The model under review builds one solid part; all positions refer to its coordinate system, in mm. A direction names the side the tool comes from. Round coordinates to 2 decimals unless told otherwise and drop trailing zeros. Loops run counter-clockwise (first coordinate to the right, second up) from the corner with the lowest first, then second, coordinate; pieces in that order, holes last. Notation, with made-up numbers: (74.5, -30.75) -> (110.5, -30.75) arc R14 ccw to (110.5, -11.75) -> close; hole circle Ø3 at (-32.75, 54.5). An arc over 180 degrees is marked (long way). Write each question's results on one line, items separated by ' | '. Start each with the question number.
Item 1: We need section B-B (z = -2). Give the boundary of the cut face in (x, y), and give its area (3 significant figures).
Item 2: Tool access review of faces 1 (the flat face through (84, 6, 0)), 2 (the flat face through (-36, 6, 0)): name each direction out of +Z, -Z, +X, -X, +Y, -Y from which nothing blocks a thin tool from reaching the whole face with its end or side.
Item 3: We need section C-C (x = 15). Give the boundary of the cut face in (y, z), and give its area (3 significant figures).
Item 4: For L1, parallel to X at y = 6.5, z = 18; L2, parallel to X at y = 2.25, z = -20.5; L3, parallel to Z at x = 13, y = 4.5, list the stretches that pass through material, from the lowest coordinate up. Write a range as from..to.
Item 5: Mouldability with a two-part tool opening along X and no side actions: class faces 3 (the flat face through (-1, 6, -23)), 4 (the flat face through (-1, 12, -24)), 5 (the flat face through (-84, 6, 0)), 6 (the cylindrical face through (-73.77, 5.92, 24.96)) as pulls with the +X half, pulls with the -X half, needs draft (parallel to the pull), parting line crosses it, or undercut.
Item 6: We need section A-A (x = -72). Give the boundary of the cut face in (y, z), and give its area (3 significant figures).
Item 7: We need section D-D (y = 4). Give the boundary of the cut face in (x, z).
from build123d import *

# Parameters (mm, degrees)
SKETCH1_W                  = 168
SKETCH1_H                  = 70
SKETCH1_R                  = 4.25
SKETCH1_W_2                = 72
SKETCH1_H_2                = 46
BRIDGE_CLAMP_EXTRUDE_DEPTH = 12


with BuildPart() as part:
    # Sketch1 → Bridge_Clamp_Extrude (new body)
    with BuildSketch(Plane(origin=(0, 0, 0), x_dir=(1, 0, 0), z_dir=(0, 1, 0))):
        Rectangle(SKETCH1_W, SKETCH1_H)
        with Locations(Location((-70, -23, 0), (0, 0, 270))):
            Circle(SKETCH1_R, mode=Mode.SUBTRACT)
        with Locations(Location((70, -23, 0), (0, 0, 270))):
            Circle(SKETCH1_R, mode=Mode.SUBTRACT)
        with Locations(Location((-70, 23, 0), (0, 0, 270))):
            Circle(SKETCH1_R, mode=Mode.SUBTRACT)
        with Locations(Location((70, 23, 0), (0, 0, 270))):
            Circle(SKETCH1_R, mode=Mode.SUBTRACT)
        Rectangle(SKETCH1_W_2, SKETCH1_H_2, mode=Mode.SUBTRACT)
    extrude(amount=BRIDGE_CLAMP_EXTRUDE_DEPTH)


solid = part.part
Here are the results:
1) outline: (-84, 0) -> (-36, 0) -> (-36, 12) -> (-84, 12) -> close; (36, 0) -> (84, 0) -> (84, 12) -> (36, 12) -> close | area: 1,150 mm2
2) face 1: +Z, -Z, +X, +Y, -Y | face 2: +Y, -Y
3) outline: (0, -35) -> (12, -35) -> (12, -23) -> (0, -23) -> close; (0, 23) -> (12, 23) -> (12, 35) -> (0, 35) -> close | area: 288 mm2
4) L1: x = -84..-36, 36..84 | L2: x = -84..-73.44, -66.56..-36, 36..66.56, 73.44..84 | L3: z = -35..-23, 23..35
5) face 3: undercut | face 4: needs draft | face 5: pulls with the -X half | face 6: undercut
6) outline: (0, -35) -> (12, -35) -> (12, -26.75) -> (0, -26.75) -> close; (0, -19.25) -> (12, -19.25) -> (12, 19.25) -> (0, 19.25) -> close; (0, 26.75) -> (12, 26.75) -> (12, 35) -> (0, 35) -> close | area: 660 mm2
7) outline: (-84, -35) -> (84, -35) -> (84, 35) -> (-84, 35) -> close; hole circle Ø8.5 at (-70, -23); hole circle Ø8.5 at (-70, 23); hole (-36, -23) -> (36, -23) -> (36, 23) -> (-36, 23) -> close; hole circle Ø8.5 at (70, -23); hole circle Ø8.5 at (70, 23)
